from build123d import *

# Parameters (mm, degrees)
BOSS_EXTRUDE1_DEPTH = 12
SKETCH2_5_R         = 17.5
CUT_EXTRUDE1_DEPTH  = 61.62435091
CUT_EXTRUDE2_DEPTH  = 61.62435091
FILLET2_R           = 1
SKETCH5_R           = 2.5
CUT_EXTRUDE3_DEPTH  = 20
SKETCH6_R           = 2.5
CUT_EXTRUDE4_DEPTH  = 20
CUT_EXTRUDE5_DEPTH  = 20


with BuildPart() as part:
    # Sketch2 → Boss-Extrude1 (new body)
    with BuildSketch(Plane.XY):
        with BuildLine():
            Line((-16.716052914, -48.420796926), (-10.73162709, -42.058723264))
            Line((-10.73162709, -42.058723264), (-4.73162709, -42.058723264))
            Line((-4.73162709, -42.058723264), (-1.004945592, -49.030501572))
            Line((-1.004945592, -49.030501572), (17.713759132, -45.729888885))
            Line((17.713759132, -45.729888885), (23.759018728, -3.392495999))
            ThreePointArc((23.759018728, -3.392495999), (23.58484248, 4.444682801), (20.894470269, 11.807671751))
            Line((20.894470269, 11.807671751), (1.412805817, 46.281788856))
            Line((1.412805817, 46.281788856), (-17.156907259, 43.007447417))
            Line((-17.156907259, 43.007447417), (-20.719877005, 4.022649671))
            Line((-20.719877005, 4.022649671), (-33.575613753, -38.686924938))
            Line((-33.575613753, -38.686924938), (-16.716052914, -48.420796926))
        make_face()
    extrude(amount=BOSS_EXTRUDE1_DEPTH)

    # Sketch2_5 → Cut-Extrude1 (cut, through all)
    with BuildSketch(Plane.XY):
        Circle(SKETCH2_5_R)
    extrude(amount=CUT_EXTRUDE1_DEPTH, mode=Mode.SUBTRACT)

    # Sketch4 → Cut-Extrude2 (cut, through all)
    with BuildSketch(Plane(origin=(0, 0, 0), x_dir=(-1, 0, 0), z_dir=(0, 0, -1))):
        with BuildLine():
            ThreePointArc((12.583655507, -35.795530683), (12.483755084, -35.036711638), (12.949680911, -34.429505279))
            Line((12.949680911, -34.429505279), (23.341985756, -28.429505279))
            ThreePointArc((23.341985756, -28.429505279), (24.100804801, -28.329604857), (24.70801116, -28.795530683))
            Line((24.70801116, -28.795530683), (27.70801116, -33.991683106))
            ThreePointArc((27.70801116, -33.991683106), (27.807911582, -34.750502151), (27.341985756, -35.357708509))
            Line((27.341985756, -35.357708509), (16.949680911, -41.357708509))
            ThreePointArc((16.949680911, -41.357708509), (16.190861866, -41.457608932), (15.583655507, -40.991683106))
            Line((15.583655507, -40.991683106), (12.583655507, -35.795530683))
        make_face()
        with BuildLine():
            ThreePointArc((-10.230917355, -28.771636769), (-11.010965186, -28.087601228), (-10.764474433, -27.079820723))
            Line((-10.764474433, -27.079820723), (-4.502269642, -20.815871366))
            ThreePointArc((-4.502269642, -20.815871366), (-3.621416209, -20.538071906), (-2.888697749, -21.100387627))
            Line((-2.888697749, -21.100387627), (0.853453027, -29.128374794))
            ThreePointArc((0.853453027, -29.128374794), (0.740397335, -30.159683501), (-0.226561789, -30.53567458))
            Line((-0.226561789, -30.53567458), (-10.230917355, -28.771636769))
        make_face()
        with BuildLine():
            ThreePointArc((-12.990634731, -33.362157195), (-12.579403415, -32.716653329), (-11.832178801, -32.55099762))
            Line((-11.832178801, -32.55099762), (-0.014485765, -34.634775752))
            ThreePointArc((-0.014485765, -34.634775752), (0.631018102, -35.046007069), (0.796673811, -35.793231683))
            Line((0.796673811, -35.793231683), (-0.245215255, -41.702078201))
            ThreePointArc((-0.245215255, -41.702078201), (-0.656446572, -42.347582067), (-1.403671186, -42.513237776))
            Line((-1.403671186, -42.513237776), (-13.221364222, -40.429459644))
            ThreePointArc((-13.221364222, -40.429459644), (-13.866868089, -40.018228328), (-14.032523797, -39.271003713))
            Line((-14.032523797, -39.271003713), (-12.990634731, -33.362157195))
        make_face()
        with BuildLine():
            Line((-0.814864543, 29.347220961), (2.927286233, 21.319233794))
            ThreePointArc((2.927286233, 21.319233794), (3.660004693, 20.756918074), (4.540858126, 21.034717534))
            Line((4.540858126, 21.034717534), (10.803062917, 27.29866689))
            ThreePointArc((10.803062917, 27.29866689), (11.04955367, 28.306447396), (10.269505839, 28.990482936))
            Line((10.269505839, 28.990482936), (0.265150273, 30.754520747))
            ThreePointArc((0.265150273, 30.754520747), (-0.701808851, 30.378529668), (-0.814864543, 29.347220961))
        make_face()
        with BuildLine():
            ThreePointArc((12.855575038, 32.59619561), (12.444343721, 31.950691743), (11.697119107, 31.785036034))
            Line((11.697119107, 31.785036034), (-0.120573929, 33.868814166))
            ThreePointArc((-0.120573929, 33.868814166), (-0.766077796, 34.280045483), (-0.931733505, 35.027270097))
            Line((-0.931733505, 35.027270097), (0.110155561, 40.936116615))
            ThreePointArc((0.110155561, 40.936116615), (0.521386878, 41.581620482), (1.268611492, 41.747276191))
            Line((1.268611492, 41.747276191), (13.086304528, 39.663498059))
            ThreePointArc((13.086304528, 39.663498059), (13.731808395, 39.252266742), (13.897464104, 38.505042128))
            Line((13.897464104, 38.505042128), (12.855575038, 32.59619561))
        make_face()
        with BuildLine():
            Line((11.63426972, -18.423588462), (20.696347848, -23.601642201))
            ThreePointArc((20.696347848, -23.601642201), (21.200226386, -24.467658925), (20.70022889, -25.335922163))
            Line((20.70022889, -25.335922163), (11.591437777, -30.594885164))
            ThreePointArc((11.591437777, -30.594885164), (10.589501007, -30.593764079), (10.091447793, -29.724384103))
            Line((10.091447793, -29.724384103), (10.138160777, -19.287367363))
            ThreePointArc((10.138160777, -19.287367363), (10.638150761, -18.425817617), (11.63426972, -18.423588462))
        make_face()
    extrude(amount=-CUT_EXTRUDE2_DEPTH, mode=Mode.SUBTRACT)

    # Fillet2
    fillet2_edges = [part.edges().sort_by_distance(p)[0] for p in [
        (-16.716052914, -48.420796926, 6),
        (-33.575613753, -38.686924938, 6),
        (-17.156907259, 43.007447417, 6),
        (1.412805817, 46.281788856, 6),
        (17.713759132, -45.729888885, 6),
        (-1.004945592, -49.030501572, 6),
        (-4.73162709, -42.058723264, 6),
        (-10.73162709, -42.058723264, 6),
    ]]
    fillet(fillet2_edges, radius=FILLET2_R)

    # Sketch5 → Cut-Extrude3 (cut)
    with BuildSketch(Plane(origin=(8.35440677, -47.380195228, 0), x_dir=(0.9848077530122075, 0.17364817766693383, 0), z_dir=(0.17364817766693386, -0.9848077530122076, 0))):
        with Locations((0, 6)):
            Circle(SKETCH5_R)
    extrude(amount=-CUT_EXTRUDE3_DEPTH, mode=Mode.SUBTRACT)

    # Sketch6 → Cut-Extrude4 (cut)
    with BuildSketch(Plane(origin=(-25.145833333, -43.553860932, 0), x_dir=(0.86602540378444, -0.4999999999999975, 0), z_dir=(-0.4999999999999975, -0.86602540378444, 0))):
        with Locations(Location((0, 6, 0), (0, 0, 180))):
            Circle(SKETCH6_R)
    extrude(amount=-CUT_EXTRUDE4_DEPTH, mode=Mode.SUBTRACT)

    # Sketch7 → Cut-Extrude5 (cut)
    with BuildSketch(Plane(origin=(-7.872050721, 44.644618137, 0), x_dir=(0.9848077530122087, 0.17364817766692725, 0), z_dir=(-0.17364817766692725, 0.9848077530122087, 0))):
        with BuildLine():
            ThreePointArc((2.528573577, -6), (0.772337028, -3.613199646), (-2.028879167, -4.579828106))
            Line((-2.028879167, -4.579828106), (2.08602632, -7.420171894))
            ThreePointArc((2.08602632, -7.420171894), (2.41537393, -6.743763451), (2.528573577, -6))
        make_face()
        with BuildLine():
            Line((2.08602632, -7.420171894), (-2.028879167, -4.579828106))
            ThreePointArc((-2.028879167, -4.579828106), (-1.391598318, -8.057452743), (2.08602632, -7.420171894))
        make_face()
    extrude(amount=-CUT_EXTRUDE5_DEPTH, mode=Mode.SUBTRACT)


solid = part.part
Geometry: final body of the model. Coordinates: model frame, mm. A direction names the side the tool comes from. Give positions to 0.01 mm unless a question says otherwise; leave off trailing zeros. Write each loop counter-clockwise with the first axis right and the second up, starting at its lowest first coordinate (ties: lowest second). Pieces come first, ordered by that corner, then holes.
(1) Cut plane B-B, the plane z = 2. Give the number of separate pieces and of enclosed holes in the cut face, then the cut area to 3 significant figures.
(2) Ray query, line 1 (Y direction, x = 12, z = 3.75); line 2 (X direction, y = 0, z = 9.5); line 3 (Y direction, x = -1.5, z = 9). Return the intervals inside material, ascending.
(3) Cut plane A-A, the plane y = 0. Return loops of the section in (x, z), then the cut area to 3 significant figures.
(4) Access query for faces 4 (the flat face through (-2.92, -45.45, 5.92)), 5 (the cylindrical face through (5.26, -31.71, 8.48)), 6 (the flat face through (-0.283, -38.706, 5.916)). Directions: +Z, -Z, +X, -X, +Y, -Y. A direction counts if a zero-diameter tool reaches every point of the face in a straight line with its end or side. Return the directions, or none.
(5) Cut plane C-C, the plane x = -29. Return loops of the section in (y, z), then the cut area to 3 significant figures.
(6) First-contact query: P1, Ø8, axis at x = 13.5, y = 36, coming from the -Z side; P2, Ø3, axis at x = -6.5, z = 8.5, coming from the +Y side; P3, Ø5.5, axis at x = -8.5, z = 5, coming from the -Y side. Flat tips, straight axial feed; report the tip coordinate or a pass-through.
(7) Mould query, pull axis X, two halves, no side actions, for faces 1 (the cylindrical face through (11.006, -28.102, 5.916)), 2 (the flat face through (-18, -1, 0)), 3 (the flat face through (-18.95, 23.4, 5.92)). Classes: released by +X, released by -X, zero draft, split by the parting line, or undercut.
Values follow:
1. separate pieces: 1
1. enclosed holes: 7
1. area: 2,230 mm2
2. line 1: y = -46.74 to -40.64, -32.54 to -12.74, 12.74 to 27.55
2. line 2: x = -21.93 to -17.5, 17.5 to 24
2. line 3: y = -48.1 to -17.44, 17.44 to 24.38, 30.54 to 33.58, 41.71 to 45.77
3. outline: (-21.93, 0) - (-17.5, 0) - (-17.5, 12) - (-21.93, 12) - close; (17.5, 0) - (24, 0) - (24, 12) - (17.5, 12) - close
3. area: 131 mm2
4. face 4: +Z, -Z, -Y
4. face 5: none
4. face 6: +Z, -Z
5. outline: (-41.33, 0) - (-23.49, 0) - (-23.49, 12) - (-41.33, 12) - close
5. area: 214 mm2
6. P1: passes through
6. P2: stops at y = 45.15
6. P3: stops at y = -42.61
7. face 1: undercut
7. face 2: zero draft
7. face 3: released by -X
